Source: CAD feature listing. Evaluate the final solid. Frame: model axes, mm. Coordinates: 2 decimals unless noted, no trailing zeros. Loops run counter-clockwise (first coordinate to the right, second up) from the corner with the lowest first, then second, coordinate; pieces in that order, holes last.
Item 1: Section query D-D, the plane y = 2.7. State how many separate pieces and enclosed holes the cut face has, then the cut area to 3 significant figures.
Item 2: Section query C-C, the plane z = 59. Return the cut outline in (x, y), then the cut area to 3 significant figures.
Item 3: Line query: probe 1 along X at (y, z) = (2.75, -11); probe 2 along X at (y, z) = (2.1, 2); probe 3 along X at (y, z) = (1.35, 95). Output: solid intervals per line, ascending.
Item 4: Section query B-B, the plane x = 49. Return the cut outline in (y, z), then the cut area to 3 significant figures.
Item 5: Pin query (flat end, axial travel): pin 1 Ø3 at (x, z) = (40.5, 50.5) entering from +Y. Return the tip coordinate at first contact, or that it passes through.
Item 6: Section query A-A, the plane z = -7. Return the cut outline in (x, y), then the cut area to 3 significant figures.
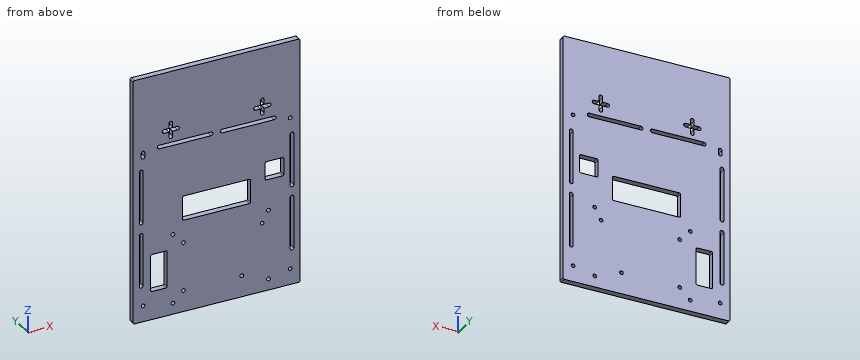
```python
from build123d import *

# Parameters (mm, degrees)
BOSS_EXTRUDE1_DEPTH = 5
CUT_EXTRUDE1_DEPTH  = 5
CUT_EXTRUDE2_DEPTH  = 5
SKETCH5_R           = 1.5
CUT_EXTRUDE3_DEPTH  = 5
CUT_EXTRUDE4_DEPTH  = 5
SKETCH6_R           = 1.5
CUT_EXTRUDE5_DEPTH  = 5
SKETCH7_R           = 1.5
CUT_EXTRUDE6_DEPTH  = 10


with BuildPart() as part:
    # Sketch1 → Boss-Extrude1 (new body)
    with BuildSketch(Plane(origin=(0, 0, 0), x_dir=(1, 0, 0), z_dir=(0, 1, 0))):
        with BuildLine():
            Line((-67.442622951, -147.745901639), (65.557377049, -147.745901639))
            ThreePointArc((65.557377049, -147.745901639), (66.26448383, -147.453008421), (66.557377049, -146.745901639))
            Line((66.557377049, -146.745901639), (66.557377049, 51.254098361))
            ThreePointArc((66.557377049, 51.254098361), (66.26448383, 51.961205142), (65.557377049, 52.254098361))
            Line((65.557377049, 52.254098361), (-67.442622951, 52.254098361))
            ThreePointArc((-67.442622951, 52.254098361), (-68.149729732, 51.961205142), (-68.442622951, 51.254098361))
            Line((-68.442622951, 51.254098361), (-68.442622951, -146.745901639))
            ThreePointArc((-68.442622951, -146.745901639), (-68.149729732, -147.453008421), (-67.442622951, -147.745901639))
        make_face()
    extrude(amount=BOSS_EXTRUDE1_DEPTH)

    # Sketch2 → Cut-Extrude1 (cut)
    with BuildSketch(Plane(origin=(0, 5, 0), x_dir=(1, 0, 0), z_dir=(0, 1, 0))):
        with BuildLine():
            Line((58.557377049, -71.245901639), (58.557377049, -29.245901639))
            ThreePointArc((58.557377049, -29.245901639), (60.057377049, -27.745901639), (61.557377049, -29.245901639))
            Line((61.557377049, -29.245901639), (61.557377049, -71.245901639))
            ThreePointArc((61.557377049, -71.245901639), (60.057377049, -72.745901639), (58.557377049, -71.245901639))
        make_face()
        with BuildLine():
            Line((58.557377049, -19.245901639), (58.557377049, 22.754098361))
            ThreePointArc((58.557377049, 22.754098361), (60.057377049, 24.254098361), (61.557377049, 22.754098361))
            Line((61.557377049, 22.754098361), (61.557377049, -19.245901639))
            ThreePointArc((61.557377049, -19.245901639), (60.057377049, -20.745901639), (58.557377049, -19.245901639))
        make_face()
        with BuildLine():
            Line((-60.442622951, -71.245901639), (-60.442622951, -29.245901639))
            ThreePointArc((-60.442622951, -29.245901639), (-61.942622951, -27.745901639), (-63.442622951, -29.245901639))
            Line((-63.442622951, -29.245901639), (-63.442622951, -71.245901639))
            ThreePointArc((-63.442622951, -71.245901639), (-61.942622951, -72.745901639), (-60.442622951, -71.245901639))
        make_face()
        with BuildLine():
            Line((-60.442622951, -19.245901639), (-60.442622951, 22.754098361))
            ThreePointArc((-60.442622951, 22.754098361), (-61.942622951, 24.254098361), (-63.442622951, 22.754098361))
            Line((-63.442622951, 22.754098361), (-63.442622951, -19.245901639))
            ThreePointArc((-63.442622951, -19.245901639), (-61.942622951, -20.745901639), (-60.442622951, -19.245901639))
        make_face()
    extrude(amount=-CUT_EXTRUDE1_DEPTH, mode=Mode.SUBTRACT)

    # Sketch3 → Cut-Extrude2 (cut)
    with BuildSketch(Plane(origin=(0, 5, 0), x_dir=(1, 0, 0), z_dir=(0, 1, 0))):
        with BuildLine():
            Line((-47.442622951, -86.545901639), (-5.442622951, -86.545901639))
            ThreePointArc((-5.442622951, -86.545901639), (-3.942622951, -88.045901639), (-5.442622951, -89.545901639))
            Line((-5.442622951, -89.545901639), (-47.442622951, -89.545901639))
            ThreePointArc((-47.442622951, -89.545901639), (-48.942622951, -88.045901639), (-47.442622951, -86.545901639))
        make_face()
        with BuildLine():
            Line((3.557377049, -86.545901639), (45.557377049, -86.545901639))
            ThreePointArc((45.557377049, -86.545901639), (47.057377049, -88.045901639), (45.557377049, -89.545901639))
            Line((45.557377049, -89.545901639), (3.557377049, -89.545901639))
            ThreePointArc((3.557377049, -89.545901639), (2.057377049, -88.045901639), (3.557377049, -86.545901639))
        make_face()
    extrude(amount=-CUT_EXTRUDE2_DEPTH, mode=Mode.SUBTRACT)

    # Sketch5 → Cut-Extrude3 (cut)
    with BuildSketch(Plane(origin=(0, 5, 0), x_dir=(1, 0, 0), z_dir=(0, 1, 0))):
        with Locations(Location((58.557377049, -84.745901639, 0), (0, 0, 270))):
            Circle(SKETCH5_R)
        with Locations(Location((58.557377049, 39.254098361, 0), (0, 0, 90))):
            Circle(SKETCH5_R)
        with Locations(Location((-60.442622951, 39.254098361, 0), (0, 0, 270))):
            Circle(SKETCH5_R)
        with BuildLine():
            Line((-58.942622951, -83.068904194), (-58.942622951, -86.422899085))
            ThreePointArc((-58.942622951, -86.422899085), (-60.442622951, -87.922899085), (-61.942622951, -86.422899085))
            Line((-61.942622951, -86.422899085), (-61.942622951, -83.068904194))
            ThreePointArc((-61.942622951, -83.068904194), (-60.442622951, -81.568904194), (-58.942622951, -83.068904194))
        make_face()
    extrude(amount=-CUT_EXTRUDE3_DEPTH, mode=Mode.SUBTRACT)

    # Sketch4 → Cut-Extrude4 (cut)
    with BuildSketch(Plane(origin=(0, 5, 0), x_dir=(1, 0, 0), z_dir=(0, 1, 0))):
        with BuildLine():
            Line((-27.442622951, -22.745901639), (25.557377049, -22.745901639))
            ThreePointArc((25.557377049, -22.745901639), (26.26448383, -23.038794858), (26.557377049, -23.745901639))
            Line((26.557377049, -23.745901639), (26.557377049, -41.745901639))
            ThreePointArc((26.557377049, -41.745901639), (26.26448383, -42.453008421), (25.557377049, -42.745901639))
            Line((25.557377049, -42.745901639), (-27.442622951, -42.745901639))
            ThreePointArc((-27.442622951, -42.745901639), (-28.149729732, -42.453008421), (-28.442622951, -41.745901639))
            Line((-28.442622951, -41.745901639), (-28.442622951, -23.745901639))
            ThreePointArc((-28.442622951, -23.745901639), (-28.149729732, -23.038794858), (-27.442622951, -22.745901639))
        make_face()
    extrude(amount=-CUT_EXTRUDE4_DEPTH, mode=Mode.SUBTRACT)

    # Sketch6 → Cut-Extrude5 (cut)
    with BuildSketch(Plane(origin=(0, 5, 0), x_dir=(1, 0, 0), z_dir=(0, 1, 0))):
        with Locations(Location((-36.251799608, 43.183284391, 0), (0, 0, 270))):
            Circle(SKETCH6_R)
        with Locations(Location((-36.251799608, -13.337715609, 0), (0, 0, 270))):
            Circle(SKETCH6_R)
        with Locations(Location((41.030032564, -13.337715609, 0), (0, 0, 270))):
            Circle(SKETCH6_R)
        with Locations(Location((41.030032564, 43.183284391, 0), (0, 0, 270))):
            Circle(SKETCH6_R)
        with BuildLine():
            Line((-53.327467893, 29.269104752), (-42.086468598, 29.269104752))
            ThreePointArc((-42.086468598, 29.269104752), (-41.379361817, 28.976211533), (-41.086468598, 28.269104752))
            Line((-41.086468598, 28.269104752), (-41.086468598, -0.204578889))
            ThreePointArc((-41.086468598, -0.204578889), (-41.379361817, -0.911685671), (-42.086468598, -1.204578889))
            Line((-42.086468598, -1.204578889), (-53.327467893, -1.204578889))
            ThreePointArc((-53.327467893, -1.204578889), (-54.034574674, -0.911685671), (-54.327467893, -0.204578889))
            Line((-54.327467893, -0.204578889), (-54.327467893, 28.269104752))
            ThreePointArc((-54.327467893, 28.269104752), (-54.034574674, 28.976211533), (-53.327467893, 29.269104752))
        make_face()
        with BuildLine():
            Line((39.416322558, -38.655645532), (52.416322558, -38.655645532))
            ThreePointArc((52.416322558, -38.655645532), (53.123429339, -38.948538751), (53.416322558, -39.655645532))
            Line((53.416322558, -39.655645532), (53.416322558, -52.655645532))
            ThreePointArc((53.416322558, -52.655645532), (53.123429339, -53.362752313), (52.416322558, -53.655645532))
            Line((52.416322558, -53.655645532), (39.416322558, -53.655645532))
            ThreePointArc((39.416322558, -53.655645532), (38.709215777, -53.362752313), (38.416322558, -52.655645532))
            Line((38.416322558, -52.655645532), (38.416322558, -39.655645532))
            ThreePointArc((38.416322558, -39.655645532), (38.709215777, -38.948538751), (39.416322558, -38.655645532))
        make_face()
        with BuildLine():
            Line((37.557377049, -94.245901639), (37.557377049, -98.245901639))
            Line((37.557377049, -98.245901639), (41.557377049, -98.245901639))
            ThreePointArc((41.557377049, -98.245901639), (43.057377049, -99.745901639), (41.557377049, -101.245901639))
            Line((41.557377049, -101.245901639), (37.557377049, -101.245901639))
            Line((37.557377049, -101.245901639), (37.557377049, -105.245901639))
            ThreePointArc((37.557377049, -105.245901639), (36.057377049, -106.745901639), (34.557377049, -105.245901639))
            Line((34.557377049, -105.245901639), (34.557377049, -101.245901639))
            Line((34.557377049, -101.245901639), (30.557377049, -101.245901639))
            ThreePointArc((30.557377049, -101.245901639), (29.057377049, -99.745901639), (30.557377049, -98.245901639))
            Line((30.557377049, -98.245901639), (34.557377049, -98.245901639))
            Line((34.557377049, -98.245901639), (34.557377049, -94.245901639))
            ThreePointArc((34.557377049, -94.245901639), (36.057377049, -92.745901639), (37.557377049, -94.245901639))
        make_face()
        with BuildLine():
            Line((-43.442622951, -98.245901639), (-39.442622951, -98.245901639))
            Line((-39.442622951, -98.245901639), (-39.442622951, -94.245901639))
            ThreePointArc((-39.442622951, -94.245901639), (-37.942622951, -92.745901639), (-36.442622951, -94.245901639))
            Line((-36.442622951, -94.245901639), (-36.442622951, -98.245901639))
            Line((-36.442622951, -98.245901639), (-32.442622951, -98.245901639))
            ThreePointArc((-32.442622951, -98.245901639), (-30.942622951, -99.745901639), (-32.442622951, -101.245901639))
            Line((-32.442622951, -101.245901639), (-36.442622951, -101.245901639))
            Line((-36.442622951, -101.245901639), (-36.442622951, -105.245901639))
            ThreePointArc((-36.442622951, -105.245901639), (-37.942622951, -106.745901639), (-39.442622951, -105.245901639))
            Line((-39.442622951, -105.245901639), (-39.442622951, -101.245901639))
            Line((-39.442622951, -101.245901639), (-43.442622951, -101.245901639))
            ThreePointArc((-43.442622951, -101.245901639), (-44.942622951, -99.745901639), (-43.442622951, -98.245901639))
        make_face()
    extrude(amount=-CUT_EXTRUDE5_DEPTH, mode=Mode.SUBTRACT)

    # Sketch7 → Cut-Extrude6 (cut)
    with BuildSketch(Plane(origin=(0, 5, 0), x_dir=(1, 0, 0), z_dir=(0, 1, 0))):
        with Locations(Location((-27.742619724, -4.439577259, 0), (0, 0, 270))):
            Circle(SKETCH7_R)
        with Locations(Location((35.925380276, -3.999577259, 0), (0, 0, 270))):
            Circle(SKETCH7_R)
        with Locations(Location((-27.742619724, 34.937422741, 0), (0, 0, 270))):
            Circle(SKETCH7_R)
        with Locations(Location((19.434380276, 34.937422741, 0), (0, 0, 270))):
            Circle(SKETCH7_R)
    extrude(amount=-CUT_EXTRUDE6_DEPTH, mode=Mode.SUBTRACT)


solid = part.part
```
Verdict:
1. separate pieces: 1
1. enclosed holes: 23
1. area: 24,200 mm2
2. outline: (-68.44, 0) - (-63.44, 0) - (-63.44, 5) - (-68.44, 5) - close; (-60.44, 0) - (58.56, 0) - (58.56, 5) - (-60.44, 5) - close; (61.56, 0) - (66.56, 0) - (66.56, 5) - (61.56, 5) - close
2. area: 645 mm2
3. probe 1: x = -68.44 to -63.44, -60.44 to -54.33, -41.09 to 58.56, 61.56 to 66.56
3. probe 2: x = -68.44 to -63.44, -60.44 to 58.56, 61.56 to 66.56
3. probe 3: x = -68.44 to -39.44, -36.44 to 34.56, 37.56 to 66.56
4. outline: (0, -52.25) - (5, -52.25) - (5, 38.66) - (0, 38.66) - close; (0, 53.66) - (5, 53.66) - (5, 147.75) - (0, 147.75) - close
4. area: 925 mm2
5. pin 1: passes through
6. outline: (-68.44, 0) - (-63.44, 0) - (-63.44, 5) - (-68.44, 5) - close; (-60.44, 0) - (-54.33, 0) - (-54.33, 5) - (-60.44, 5) - close; (-41.09, 0) - (58.56, 0) - (58.56, 5) - (-41.09, 5) - close; (61.56, 0) - (66.56, 0) - (66.56, 5) - (61.56, 5) - close
6. area: 579 mm2
